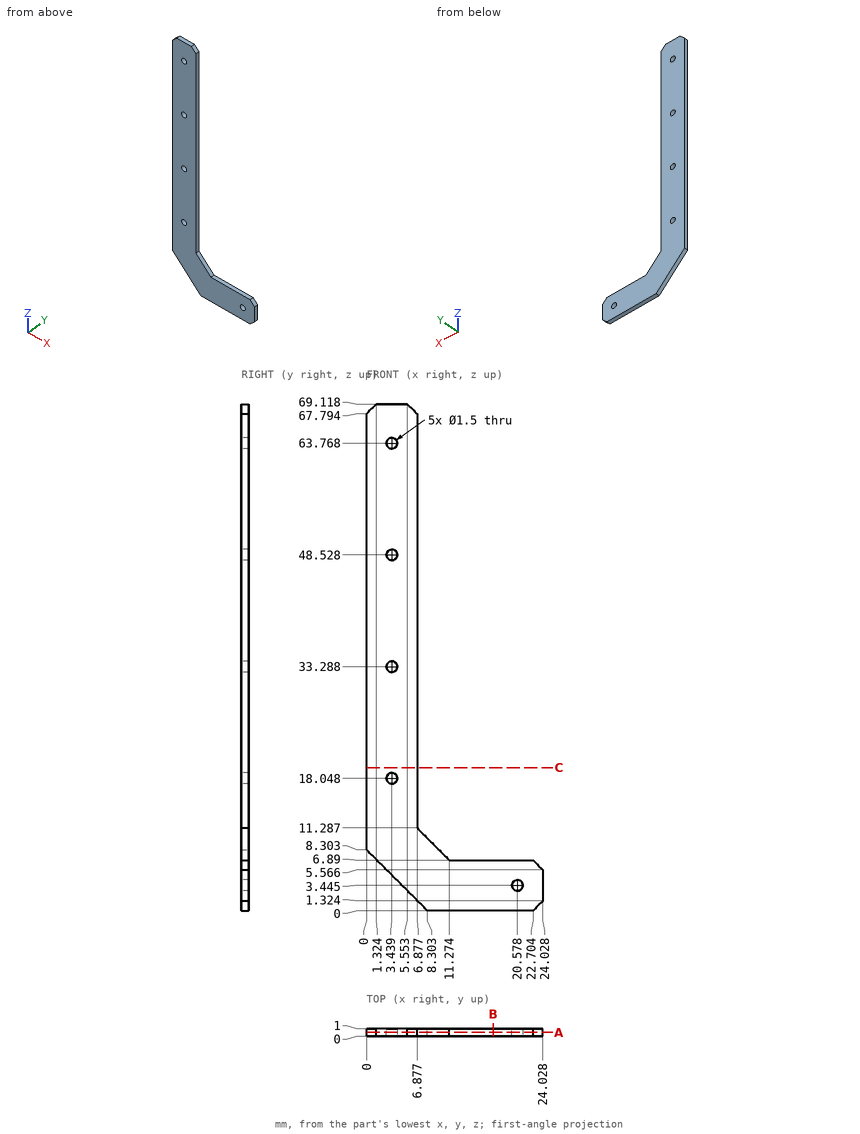
The drawing under review shows one solid part. Ordinate dimensions are in mm from its lowest x, y, z. Round coordinates to 2 decimals unless told otherwise and drop trailing zeros. Order: outer loops, then holes, each group sorted by start corner. A loop starts at its lowest first (then second) coordinate and runs counter-clockwise, first axis right, second up. Notation, with made-up numbers: (70, -37) -> (102, -37) arc R25 ccw to (102, -22) -> close; hole circle Ø6 at (79, 50). An arc over 180 degrees is marked (long way). Use a Markdown table: item, result.
Q1. We need section A-A on y = 0.5. State how many separate pieces and enclosed holes the cut face has.
Values:
| item | result |
|---|---|
| separate pieces | 1 |
| enclosed holes | 5 |
Q2. We need section B-B on x = 17.25. Write out the cut boundary in (y, z).
Values:
| item | result |
|---|---|
| outline | (0, 0) -> (1, 0) -> (1, 6.89) -> (0, 6.89) -> close |
Q3. For line 1 (Z direction, x = 20.5, y = 0.75); line 2 (Z direction, x = 15.5, y = 0.65); line 3 (X direction, y = 0.4, z = 48.5), list the stretches that pass through material, from the lowest coordinate up.
Values:
| item | result |
|---|---|
| line 1 | z = 0 to 2.7, 4.19 to 6.89 |
| line 2 | z = 0 to 6.89 |
| line 3 | x = 0 to 2.69, 4.19 to 6.88 |
Q4. We need section C-C on z = 19.5. Write out the cut boundary in (x, y).
Values:
| item | result |
|---|---|
| outline | (0, 0) -> (6.88, 0) -> (6.88, 1) -> (0, 1) -> close |
